For this review, take the finished solid that the model builds, in its own axes (mm). A direction names the side the tool comes from. Give positions to 0.01 mm unless a question says otherwise; leave off trailing zeros. Write each loop counter-clockwise with the first axis right and the second up, starting at its lowest first coordinate (ties: lowest second). Pieces come first, ordered by that corner, then holes.
1) We need section B-B on y = 0.5. Give the boundary of the cut face in (x, z).
2) Draft analysis for pull direction Y (two halves, no side actions). For faces 1 (the face through (14.2, 2, 2)), 2 (the face through (-9.822, 2.008, 6.859)), 3 (the face through (0, 4, 5)), state which applies: pulls with the +Y half, pulls with the -Y half, needs draft (parallel to the pull), parting line crosses it, or undercut.
3) Machinability: for faces 4 (the face through (-17, 2, 7)), 5 (the face through (-10.813, 1.376, 3.219)), 6 (the face through (15.25, 2.38, 8.24)), 7 (the face through (17.4, 2, 7)), 8 (the face through (0, 2, 0)), which of the approach directions +Z, -Z, +X, -X, +Y, -Y give a long, thin tool a straight path to every point of the face, cutting with its end or side? Answer none if there is none.
4) For P1, Ø5, axis at x = 1.5, z = 8, coming from the -Y side; P2, Ø2, axis at y = 2, z = 1.5, coming from the +X side; P3, Ø0.6, axis at x = 17.5, y = 1, coming from the -Z side; P4, Ø1.8, axis at x = 10, y = 2, coming from the -Z side, all flat-tipped, find the tip position at first contact; note any pin that passes through.
5) We need section A-A on z = 8. Give the boundary of the cut face in (x, y) (3 decimals), and give its area (3 significant figures).
6) Wall thickness on line 1 along Y through (x, z) = (-10, 3.5) (3 decimals); line 2 along X through (y, z) = (2, 1.5) (3 decimals); line 3 along X through (y, z) = (1.2, 1.5): over which ranges is each line inside the solid? List them lowest first.
7) We need section C-C on z = 2.5. Give the boundary of the cut face in (x, y) (3 decimals), and give its area (3 significant figures).
from build123d import *

# Parameters (mm, degrees)
SKETCH1_W                    = 36.4
SKETCH1_H                    = 9.8
BOSS_EXTRUDE1_DEPTH          = 4
SKETCH2_W                    = 4
SKETCH2_H                    = 6.999999999
CUT_EXTRUDE1_DEPTH           = 22.05421573
SKETCH3_W                    = 4
SKETCH3_H                    = 6.999999999
CUT_EXTRUDE2_DEPTH           = 22.05421573
M2_5X0_45_TAPPED_HOLE1_D     = 2.05
M2_5X0_45_TAPPED_HOLE1_DEPTH = 6.35
M2_5X0_45_TAPPED_HOLE1_TIP   = 0.615882135
M2_5X0_45_TAPPED_HOLE2_D     = 2.05
FILLET1_R                    = 2


with BuildPart() as part:
    # Sketch1 → Boss-Extrude1 (new body)
    with BuildSketch(Plane(origin=(0, 4, 0), x_dir=(1, 0, 0), z_dir=(0, 1, 0))):
        with Locations((0, -4.9)):
            Rectangle(SKETCH1_W, SKETCH1_H)
    extrude(amount=-BOSS_EXTRUDE1_DEPTH)

    # Sketch2 → Cut-Extrude1 (cut, through all)
    with BuildSketch(Plane.XZ):
        with Locations((-16.2, 3.5)):
            Rectangle(SKETCH2_W, SKETCH2_H)
    extrude(amount=-CUT_EXTRUDE1_DEPTH, mode=Mode.SUBTRACT)

    # Sketch3 → Cut-Extrude2 (cut, through all)
    with BuildSketch(Plane.XZ):
        with Locations((16.2, 3.5)):
            Rectangle(SKETCH3_W, SKETCH3_H)
    extrude(amount=-CUT_EXTRUDE2_DEPTH, mode=Mode.SUBTRACT)

    # M2.5x0.45 Tapped Hole1
    with Locations(Plane(origin=(0, 0, 0), x_dir=(-1, 0, 0), z_dir=(0, 0, -1))):
        with Locations((10, 2), (-10, 2)):
            Hole(M2_5X0_45_TAPPED_HOLE1_D / 2, depth=M2_5X0_45_TAPPED_HOLE1_DEPTH)
            with Locations((0, 0, -(M2_5X0_45_TAPPED_HOLE1_DEPTH + M2_5X0_45_TAPPED_HOLE1_TIP / 2))):  # 118° drill point
                Cone(0, M2_5X0_45_TAPPED_HOLE1_D / 2, M2_5X0_45_TAPPED_HOLE1_TIP, mode=Mode.SUBTRACT)

    # M2.5x0.45 Tapped Hole2 (through all)
    with Locations(Plane.XY.offset(9.8)):
        with Locations((16.2, 2)):
            Hole(M2_5X0_45_TAPPED_HOLE2_D / 2)

    # Fillet1
    # the kernel refuses this fillet: 2 mm, written as the material it adds along each edge
    with BuildSketch(Plane(origin=(-14.2, 0, 6.999999999), x_dir=(0, 0, -1), z_dir=(0, 1, 0))) as fillet1_piece_1:
        with BuildLine():
            CenterArc((FILLET1_R, FILLET1_R), FILLET1_R, 180, 90)
            Line((0, FILLET1_R), (0, 0))
            Line((0, 0), (FILLET1_R, 0))
        make_face()
    extrude(amount=4)
    with BuildSketch(Plane(origin=(14.2, 0, 6.999999999), x_dir=(0, 0, -1), z_dir=(0, 1, 0))) as fillet1_piece_2_section:
        with BuildLine():
            CenterArc((FILLET1_R, -FILLET1_R), FILLET1_R, 90, 90)
            Line((0, -FILLET1_R), (0, 0))
            Line((0, 0), (FILLET1_R, 0))
        make_face()
    fillet1_piece_2 = extrude(amount=4, mode=Mode.PRIVATE)
    fillet1_piece_2 = fillet1_piece_2 - Plane(origin=(16.2, 2, 6.528177275), x_dir=(-1, 0, 0), z_dir=(0, 0, -1)) * Cylinder(1.025, 16, mode=Mode.PRIVATE)
    add(fillet1_piece_2)


solid = part.part
Results list:
1. outline: (-18.2, 7) - (-16.2, 7) arc R2 cw to (-14.2, 5) - (-14.2, 0) - (14.2, 0) - (14.2, 5) arc R2 cw to (16.2, 7) - (18.2, 7) - (18.2, 9.8) - (-18.2, 9.8) - close
2. face 1: needs draft
2. face 2: undercut
2. face 3: pulls with the +Y half
3. face 4: -Z, -X, +Y, -Y
3. face 5: -Z
3. face 6: +Z, -Z
3. face 7: -Z, +X, +Y, -Y
3. face 8: -Z, +X, -X, +Y, -Y
4. P1: stops at y = 0
4. P2: stops at x = 14.2
4. P3: stops at z = 7
4. P4: stops at z = 6.43
5. outline: (-18.2, 0) - (18.2, 0) - (18.2, 4) - (-18.2, 4) - close; hole circle Ø2.05 at (16.2, 2)
5. area: 142 mm2
6. line 1: y = 0 to 0.975, 3.025 to 4
6. line 2: x = -14.2 to -11.025, -8.975 to 8.975, 11.025 to 14.2
6. line 3: x = -14.2 to -10.64, -9.36 to 9.36, 10.64 to 14.2
7. outline: (-14.2, 0) - (14.2, 0) - (14.2, 4) - (-14.2, 4) - close; hole circle Ø2.05 at (-10, 2); hole circle Ø2.05 at (10, 2)
7. area: 107 mm2
